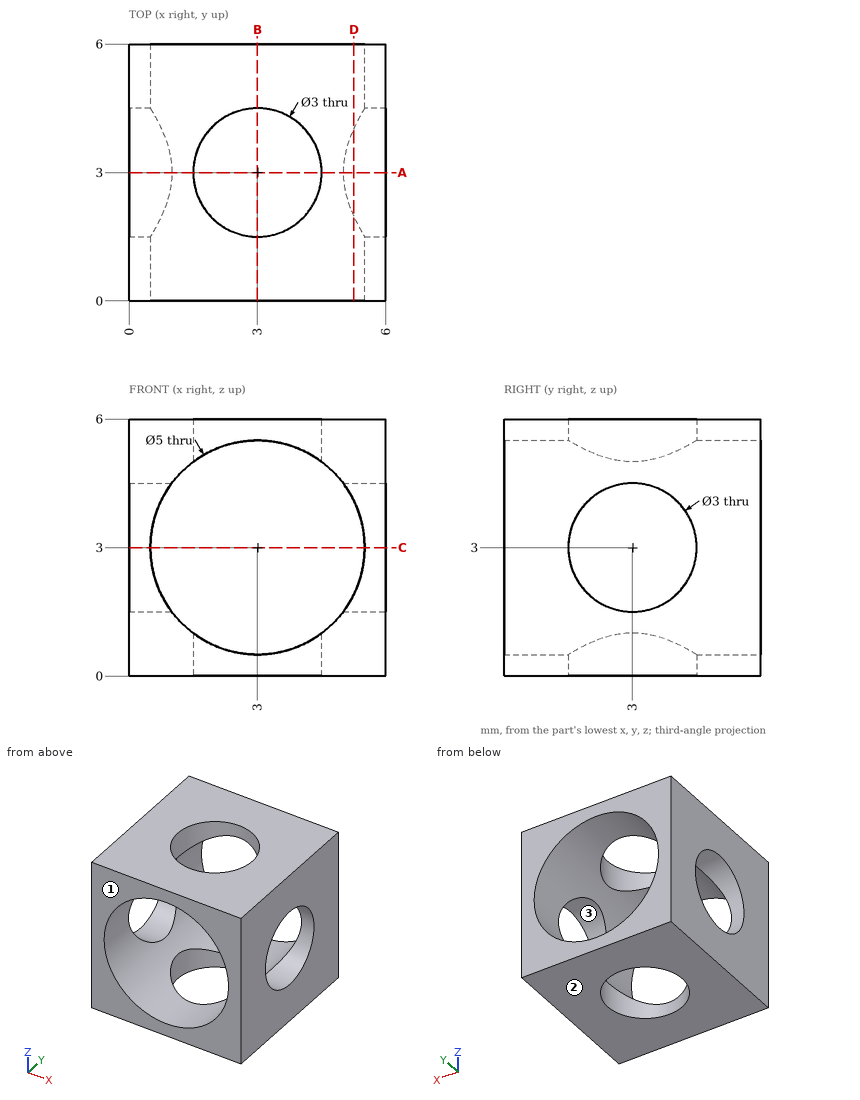
Could you check a few things on this drawing? It's one solid part, dimensions in mm from its lowest x, y, z. Give positions to 0.01 mm unless a question says otherwise; leave off trailing zeros. Order: outer loops, then holes, each group sorted by start corner. A loop starts at its lowest first (then second) coordinate and runs counter-clockwise, first axis right, second up.
1. Suppose I cut it at B-B (x = 3). Write out the boundary of the cut face in (y, z), plus the area to 3 significant figures.
Answers below:
outline: (0, 0) - (1.5, 0) - (1.5, 0.5) - (0, 0.5) - close; (0, 5.5) - (1.5, 5.5) - (1.5, 6) - (0, 6) - close; (4.5, 0) - (6, 0) - (6, 0.5) - (4.5, 0.5) - close; (4.5, 5.5) - (6, 5.5) - (6, 6) - (4.5, 6) - close
area: 3.00 mm2
2. Suppose I cut it at C-C (z = 3). Write out the boundary of the cut face in (x, y).
Answers below:
outline: (0, 0) - (0.5, 0) - (0.5, 1.5) - (0, 1.5) - close; (0, 4.5) - (0.5, 4.5) - (0.5, 6) - (0, 6) - close; (5.5, 0) - (6, 0) - (6, 1.5) - (5.5, 1.5) - close; (5.5, 4.5) - (6, 4.5) - (6, 6) - (5.5, 6) - close
3. I need wall thicknesses on L1, parallel to Y at x = 3, z = 5.55; L2, parallel to X at y = 2, z = 1.5. Which ranges of each line are inside material? Lowest first, please.
Answers below:
L1: y = 0 to 1.5, 4.5 to 6
L2: x = 0 to 1, 5 to 6
4. Thinking about a two-plate mould opening in Z: for the marked faces 1, 2 and 3, which applies, +Z half, -Z half, draft (parallel to the pull), parting line (faces both ways), or undercut?
Answers below:
face 1: draft
face 2: -Z half
face 3: undercut
5. Suppose I cut it at D-D (x = 5.25). Write out the boundary of the cut face in (y, z), plus the area to 3 significant figures.
Answers below:
outline: (0, 0) - (6, 0) - (6, 1.91) - (4.03, 1.91) arc R1.5 cw to (1.97, 1.91) - (0, 1.91) - close; (0, 4.09) - (1.97, 4.09) arc R1.5 cw to (4.03, 4.09) - (6, 4.09) - (6, 6) - (0, 6) - close
area: 21.8 mm2
6. Suppose I cut it at A-A (y = 3). Write out the boundary of the cut face in (x, z), plus the area to 3 significant figures.
Answers below:
outline: (0, 0) - (1.5, 0) - (1.5, 1) arc R2.5 cw to (1, 1.5) - (0, 1.5) - close; (0, 4.5) - (1, 4.5) arc R2.5 cw to (1.5, 5) - (1.5, 6) - (0, 6) - close; (4.5, 0) - (6, 0) - (6, 1.5) - (5, 1.5) arc R2.5 cw to (4.5, 1) - close; (4.5, 5) arc R2.5 cw to (5, 4.5) - (6, 4.5) - (6, 6) - (4.5, 6) - close
area: 8.45 mm2
7. For pin 1 (1.5 mm diameter, centred on x = 1.5, z = 4.5, fed in from -Y), with a flat end and sliding along its axis, tell me the tip position at first contact or that it passes through.
Answers below:
pin 1: stops at y = 0
